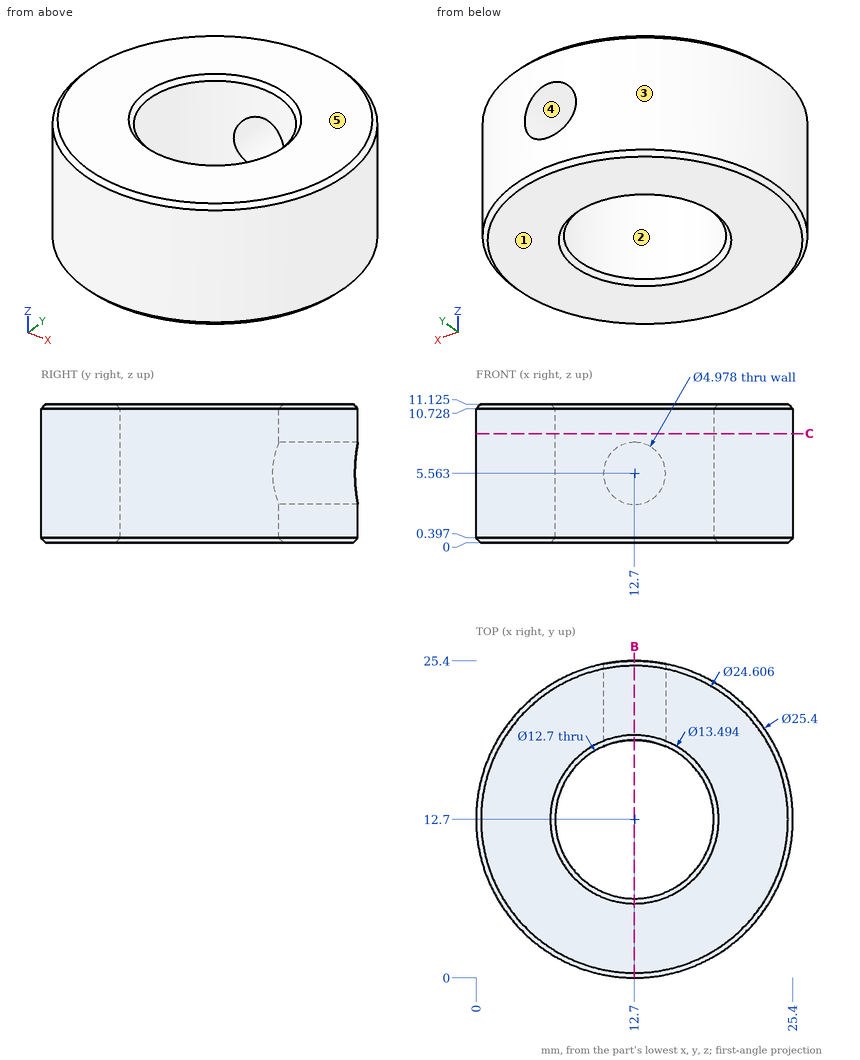
Study the drawing (mm; zero at the part's minimum x, y, z) and answer. A direction names the side the tool comes from. Give positions to 0.01 mm unless a question says otherwise; leave off trailing zeros. Write each loop counter-clockwise with the first axis right and the second up, starting at its lowest first coordinate (ties: lowest second). Pieces come first, ordered by that corner, then holes. Notation, with made-up numbers: (77.5, 78) - (124.5, 78) arc R21 cw to (124.5, 85) - close; hole circle Ø6 at (82.25, 44). An arc over 180 degrees is marked (long way). Use CSV: the item, a comma, the result in double quotes. Start each with the question number.
(1) Given P1, Ø3, axis at y = 5, z = 3, coming from the -X side; P2, Ø2, axis at x = 17, z = 6.5, coming from the +Y side; P3, Ø1.5, axis at y = 6, z = 4, coming from the -X side, each flat-ended and moving along its own axis, determine where each tip first touches the part or whether it passes through.
(2) Determine the mould class of the marked faces 1, 2 and 3 for opening direction Y: +Y half, -Y half, draft (parallel to the pull), parting line (faces both ways), or undercut.
(3) Consider line 1 along X through (y, z) = (13, 4.5); line 2 along Y through (x, z) = (12.7, 8.5); line 3 along Y through (x, z) = (12.7, 7). Determine where each line is inside the solid, lowest interval first.
(4) Find section C-C (z = 8.75). Give the vertices of the cut face in (x, y), plus the area to 3 significant figures.
(5) Find section B-B (x = 12.7). Count the separate pieces of the cut face and the enclosed holes in it, plus the area to 3 significant figures.
(6) For the marked faces 4 and 5, determine the directions among +Z, -Z, +X, -X, +Y, -Y from which every point of the face is accessible in a straight line to the end or side of a thin tool.
Findings below:
1,P1,"x = 1.62"
1,P2,"y = 24.96"
1,P3,"x = 1.48"
2,face 1,"draft"
2,face 2,"undercut"
2,face 3,"parting line"
3,line 1,"0 to 6.36, 19.04 to 25.4"
3,line 2,"0 to 6.35, 19.05 to 25.4"
3,line 3,"0 to 6.35"
4,outline,"circle Ø25.4 at (12.7, 12.7); hole circle Ø12.7 at (12.7, 12.7)"
4,area,"380 mm2"
5,separate pieces,"3"
5,enclosed holes,"0"
5,area,"109 mm2"
6,face 4,"+Y"
6,face 5,"+Z, +X, -X, +Y, -Y"
